Autodesk Inventor part; units mm, degrees
ref_plane "YZ Plane" through (0, 0, 0) normal (1, 0, 0) x (0, 1, 0)
ref_plane "XZ Plane" through (0, 0, 0) normal (0, 1, 0) x (-1, 0, 0)
ref_plane "XY Plane" through (0, 0, 0) normal (0, 0, 1) x (1, 0, 0)
sketch "Sketch1" plane through (0, 0, 0) normal (0, 1, 0) x (-1, 0, 0)
  arc A0 (-152, 0) -> (152, 0) centre (0, 100) ccw
  line L0 (0, -81.945) -> (-47.311, 0)
  line L1 (-47.311, 0) -> (47.311, 0) construction
  line L2 (47.311, 0) -> (0, -81.945)
  line L3 (0, 0) -> (68.5411, -68.5411)
  line L4 (0, 0) -> (-68.5411, -68.5411)
  line L5 (47.311, 0) -> (116.3651, -39.8684)
  line L6 (-47.311, 0) -> (-116.3651, -39.8684)
  line L7 (114.7776, -42.618) -> (48.4731, -4.3371)
  line L8 (48.4731, -4.3371) -> (0, -88.295)
  line L9 (0, -88.295) -> (-48.4731, -4.3371)
  line L10 (-48.4731, -4.3371) -> (-114.4332, -42.4192)
  line L11 (-66.0999, -70.5901) -> (0, -4.4901)
  line L12 (0, -4.4901) -> (66.2961, -70.7862)
  line L13 (116.3651, -39.8684) -> (114.7776, -42.618)
  line L14 (68.5411, -68.5411) -> (66.2961, -70.7862)
  line L15 (-66.0999, -70.5901) -> (-67.8825, -68.8075)
  line L16 (-114.4332, -42.4192) -> (-115.4867, -40.5945)
  arc A1 (-157.2837, -3.5223) -> (157.2837, -3.5223) centre (0, 100) ccw
  line L17 (157.2837, -3.5223) -> (152, 0)
  line L18 (-152, 0) -> (-157.2837, -3.5223)
  line L19 (116.3651, -39.8684) -> (113.3651, -39.8684)
  line L20 (113.3651, -39.8684) -> (113.3651, 0)
  line L21 (113.3651, 0) -> (116.3651, 0)
  line L22 (116.3651, 0) -> (116.3651, -39.8684)
  line L23 (0, 0) -> (0, -27.315) construction
  line L24 (-116.3651, -39.8684) -> (-113.3651, -39.8684)
  line L25 (-113.3651, -39.8684) -> (-113.3651, 0)
  line L26 (-113.3651, 0) -> (-116.3651, 0)
  line L27 (-116.3651, 0) -> (-116.3651, -39.8684)
  point P0 (-3.6878, -81.9077)
  point P1 (-65.3239, -69.814)
  point P2 (-30.6747, -35.1649)
  point P3 (29.994, -29.994)
  point P4 (-29.994, -29.994)
  point P5 (32.3182, -32.3182)
  point P6 (113.7344, -42.0158)
  point P7 (30.6747, -35.1649)
  point P8 (65.3239, -69.814)
  point P9 (3.6878, -81.9077)
  point P10 (-28.3505, -32.8406)
  point P11 (28.3505, -32.8406)
  point P12 (-32.3182, -32.3182)
  point P13 (-113.7344, -42.0158)
  point P14 (-113.3651, -38.1363)
  point P15 (113.3651, -38.1363)
  point P16 (0, 0)
  dimension "d0" = 152
  dimension "d1" = 152
  dimension "d2" = 100
  dimension "d3" = 0
  dimension "d4" = 45
  dimension "d8" = 3.175
  dimension "d9" = 3.175
  dimension "d10" = 6.35
  dimension "d11" = 6.35
  dimension "d12" = 3.5223
  dimension "d13" = 3.5223
  dimension "d29" = 3
  dimension "d30" = 157.2837
extrude "Extrusion1" add sketch "Sketch1" along normal mid plane 3 contours A0 L16 L10 L15 L11 L9 A1 L18 | L24 L25 L6 L0 L4 L9 L10 A0 | L27 L26 L25 L6 | L6 L25 L24 | A0 L10 L16 | L9 A0 L8 | L8 A0 L12 L14 L7 L13 L17 A1 | A0 L2 L12 L8 | L9 L11 L0 A0 | L4 L9 L11 A0 | L4 L3 L2 L12 L11 L0 | L0 L11 L9 L4 | L12 L8 L3 A0 | A0 L14 L12 | L12 L2 L3 L8 | L11 L15 A0 | L3 L2 L5 L20 L19 A0 L7 L8 | L13 L7 A0 | L19 L20 L5 | L5 L20 L21 L22
sketch "Sketch2" plane through (0, 1.5, 0) normal (0, 1, 0) x (1, 0, 0)
  line L0 (0, 0) -> (29.994, 29.994)
  line L1 (0, 0) -> (200, 0)
  line L2 (200, 0) -> (200, 200)
  line L3 (200, 200) -> (0, 200)
  line L4 (0, 200) -> (0, 0)
  dimension "d16" = 200
  dimension "d17" = 200
extrude "Extrusion2" cut sketch "Sketch2" along normal through all both and the other way through all
sketch "Sketch3" plane through (0, 1.5, 0) normal (0, 1, 0) x (1, 0, 0)
  line L0 (-29.994, 29.994) -> (0, 0)
  circle A0 centre (0, 0) radius 5
  line L1 (-157.2837, 3.5223) -> (-152, 0)
  line L2 (-47.311, 0) -> (-29.994, 29.994)
  circle A1 centre (-47.311, 0) radius 5
  line L3 (0, 81.945) -> (0, 88.295)
  circle A2 centre (0, 85.12) radius 5
  circle A3 centre (-152, 0) radius 5
  line L4 (-116.3651, 0) -> (-113.3651, 0)
  circle A4 centre (-114.8651, 0) radius 5
  dimension "d20" = 10
extrude "Circular_Mounts" add sketch "Sketch3" against normal blind 3
sketch "Sketch4" plane through (0, 1.5, 0) normal (0, 1, 0) x (1, 0, 0)
  arc A0 (-51.6411, 2.5) -> (-44.811, 4.3301) centre (-47.311, 0) ccw
  circle A1 centre (-47.311, 0) radius 4.05
  circle A2 centre (0, 0) radius 4.05
  arc A3 (-156.1603, 2.7735) -> (-149.1948, 4.1389) centre (-152, 0) ccw
  circle A4 centre (-152, 0) radius 4.05
  arc A5 (-0.9958, 80.2202) -> (-3.8953, 88.2548) centre (0, 85.12) ccw
  circle A6 centre (0, 85.12) radius 4.05
  arc A7 (-116.3651, 4.7697) -> (-113.3651, 4.7697) centre (-114.8651, 0) ccw
  circle A8 centre (-114.8651, 0) radius 4.05
  dimension "d23" = 8.1
extrude "Inserts" add sketch "Sketch4" against normal blind 7
fillet "Fillet2" radius 0.5 5 edges at (-156.05, -5.5, 0) (-51.361, -5.5, 0) (-4.05, -5.5, 0) (-4.05, -5.5, -85.12) (-118.9151, -5.5, 0)
fillet "Fillet3" radius 2 2 edges at (-156.1603, 0, -2.7735) (-157.2837, 0, -3.5223)
extrude "Extrusion5" cut sketch "Sketch4" along normal through all both and the other way through all contours A2 | A6
equation "\"d1\" = d0"
properties part number "E-Support" material "ABS Plastic"
Check sheet for the modelled part. Datum: model origin and axes. Units: mm. A direction names the side the tool comes from. Round coordinates to 2 decimals unless told otherwise and drop trailing zeros. Order: outer loops, then holes, each group sorted by start corner. A loop starts at its lowest first (then second) coordinate and runs counter-clockwise, first axis right, second up. Notation, with made-up numbers: M 73,35.25 L 111,35.25 A19 cw 111,41.25 Z; hole C 74,-35.75 d6. An arc over 180 degrees is marked long. Answer in a Markdown table with one row per item.
(1) Section check C-C on x = -9. Record the boundary of the cut face in (y, z), plus the area to 3 significant figures.
Findings:
| item | result |
|---|---|
| outline | M -1.5,-88.08 L 1.5,-88.08 L 1.5,-81.72 L -1.5,-81.72 Z; M -1.5,-72.71 L 1.5,-72.71 L 1.5,-66.36 L -1.5,-66.36 Z; M -1.5,-13.49 L 1.5,-13.49 L 1.5,-9 L -1.5,-9 Z |
| area | 51.6 mm^2 |
(2) Section check B-B on x = -88. Record the boundary of the cut face in (y, z).
Findings:
| item | result |
|---|---|
| outline | M -1.5,-66.47 L 1.5,-66.47 L 1.5,-59.25 L -1.5,-59.25 Z; M -1.5,-27.16 L 1.5,-27.16 L 1.5,-23.49 L -1.5,-23.49 Z |
(3) Set-up check for faces 4 (the flat face through (-81.854, -0.021, -23.61)), 5 (the flat face through (-152, -5.5, 0)), 6 (the cylindrical face through (-118.91, -3.23, -0.18)): record each of +Z, -Z, +X, -X, +Y, -Y from which the full face is reachable in a straight line by a thin tool's end or side.
Findings:
| item | result |
|---|---|
| face 4 | +Y, -Y |
| face 5 | +Z, -Z, +X, -X, -Y |
| face 6 | -Y |
(4) Section check A-A on z = -62. Record the boundary of the cut face in (x, y).
Findings:
| item | result |
|---|---|
| outline | M -95.97,-1.5 L -82.83,-1.5 L -82.83,1.5 L -95.97,1.5 Z; M -62,-1.5 L -57.51,-1.5 L -57.51,1.5 L -62,1.5 Z; M -15.18,-1.5 L -11.52,-1.5 L -11.52,1.5 L -15.18,1.5 Z |
(5) Draft check along X on faces 1 (the flat face through (-47, -5.5, 0)), 2 (the flat face through (-14.22, -0.02, -18.71)), 3 (the flat face through (-47.76, -0.02, -52.25)). Enter one of: +X half, -X half, draft (parallel to the pull), parting line (faces both ways), or undercut.
Findings:
| item | result |
|---|---|
| face 1 | draft |
| face 2 | +X half |
| face 3 | undercut |
(6) Gauge pin test, flat ends, axial feed: pin 1 (9.5 mm diameter, centred on x = 0, z = 0, fed in from +Y); pin 2 (2 mm diameter, centred on x = -97, z = -29, fed in from -Y); pin 3 (2.5 mm diameter, centred on y = -0.5, z = -21.5, fed in from +X); pin 4 (4 mm diameter, centred on y = -3, z = -66, fed in from +X). Record the tip position at first contact, or that the pin passes through.
Findings:
| item | result |
|---|---|
| pin 1 | stops at y = 1.5 |
| pin 2 | stops at y = -1.5 |
| pin 3 | stops at x = -15.76 |
| pin 4 | stops at x = -8.44 |
(7) Section check D-D on z = -74. Record the boundary of the cut face in (x, y).
Findings:
| item | result |
|---|---|
| outline | M -71.97,-1.5 L -53.18,-1.5 L -53.18,1.5 L -71.97,1.5 Z; M -8.25,-1.5 L -4.59,-1.5 L -4.59,1.5 L -8.25,1.5 Z |
(8) Material ranges on line 1 along Z through (x, y) = (0, 0.5); line 2 along X through (y, z) = (-0.35, 0); line 3 along Z through (x, y) = (-10, 1), recorded low to high. Write a range as from..to.
Findings:
| item | result |
|---|---|
| line 1 | z = -90.12..-89.17, -81.07..-80.12, -5..-4.05, 4.05..5 |
| line 2 | x = -157..-147, -119.87..-109.87, -52.31..-42.31, -5..-4.05, 4.05..5 |
| line 3 | z = -88.03..-81.67, -70.97..-64.62, -14.49..-10 |
